Design review of the part built by this model. Coordinates are the model's own, in mm. A direction names the side the tool comes from. Give positions to 0.01 mm unless a question says otherwise; leave off trailing zeros. Loops run counter-clockwise (first coordinate to the right, second up) from the corner with the lowest first, then second, coordinate; pieces in that order, holes last. Notation, with made-up numbers: (-7.5, -40) -> (43.5, -40) arc R22 cw to (43.5, -11) -> close; hole circle Ø9 at (-25.5, 65). An arc over 180 degrees is marked (long way). Answer in a Markdown table with one row per item. Add a question column.
(1) For faces 1 (the flat face through (22.67, -1150.66, 35.4)), 2 (the flat face through (23.09, -1150.66, 36.52)), list the 3-axis set-ups (+Z, -Z, +X, -X, +Y, -Y) from which the entire face can be reached by the end or side of a thin tool; tool diameter is ignored.
(2) For pin 1 (11 mm diameter, centred on y = -1152.5, z = 5, fed in from +X); pin 2 (5 mm diameter, centred on y = -1213, z = 2.5, fed in from -X); pin 3 (2 mm diameter, centred on x = 13, y = -358.5, fed in from +Z), all flat-tipped, find the tip position at first contact; note any pin that passes through.
(3) Consider section B-B on x = 27.5. Write out the cut boundary in (y, z).
(4) For line 1 (X direction, y = -1862.5, z = 5.5); line 2 (X direction, y = -2009.5, z = 48); line 3 (Z direction, x = 58.5, y = -665), list the stretches that pass through material, from the lowest coordinate up.
(5) Consider section A-A on y = -1767. Write out the cut boundary in (x, z).
from build123d import *

# Parameters (mm, degrees)
F1_DEPTH = 2334


with BuildPart() as f1:
    # F0 (on Front) → F1 (new body)
    with BuildSketch(Plane.XZ):
        with BuildLine():
            Line((0, 10), (0, 0))
            Line((0, 0), (1, 0))
            Line((1, 0), (1, 10))
            ThreePointArc((1, 10), (0.414214, 11.414214), (-1, 12))
            Line((-1, 12), (-13, 12))
            ThreePointArc((-13, 12), (-13.707107, 12.292893), (-14, 13))
            Line((-14, 13), (-14, 26.397954))
            ThreePointArc((-14, 26.397954), (-13.780479, 27.023135), (-13.218295, 27.373836))
            Line((-13.218295, 27.373836), (59.579564, 43.657993))
            ThreePointArc((59.579564, 43.657993), (60.703931, 44.359395), (61.142973, 45.609759))
            Line((61.142973, 45.609759), (61.142973, 53.808736))
            Line((61.142973, 53.808736), (60.142973, 53.808736))
            Line((60.142973, 53.808736), (60.142973, 45.609759))
            ThreePointArc((60.142973, 45.609759), (59.923452, 44.984577), (59.361268, 44.633876))
            Line((59.361268, 44.633876), (-14.218295, 28.17486))
            ThreePointArc((-14.218295, 28.17486), (-14.780479, 27.824159), (-15, 27.198977))
            Line((-15, 27.198977), (-15, 12))
            ThreePointArc((-15, 12), (-14.707107, 11.292893), (-14, 11))
            Line((-14, 11), (-1, 11))
            ThreePointArc((-1, 11), (-0.292893, 10.707107), (0, 10))
        make_face()
    extrude(amount=F1_DEPTH)


solid = f1.part
Values follow:
| question | item | result |
|---|---|---|
| 1 | face 1 | +X, +Y, -Y |
| 1 | face 2 | +Z, -X, +Y, -Y |
| 2 | pin 1 | x = 1 |
| 2 | pin 2 | x = 0 |
| 2 | pin 3 | z = 34.49 |
| 3 | outline | (-2334, 36.48) -> (0, 36.48) -> (0, 37.51) -> (-2334, 37.51) -> close |
| 4 | line 1 | 0 to 1 |
| 4 | line 2 | 60.14 to 61.14 |
| 4 | line 3 | 43.42 to 44.44 |
| 5 | outline | (-15, 12) arc R1 ccw to (-14, 11) -> (-1, 11) arc R1 cw to (0, 10) -> (0, 0) -> (1, 0) -> (1, 10) arc R2 ccw to (-1, 12) -> (-13, 12) arc R1 cw to (-14, 13) -> (-14, 26.4) arc R1 cw to (-13.22, 27.37) -> (59.58, 43.66) arc R2 ccw to (61.14, 45.61) -> (61.14, 53.81) -> (60.14, 53.81) -> (60.14, 45.61) arc R1 cw to (59.36, 44.63) -> (-14.22, 28.17) arc R1 ccw to (-15, 27.2) -> close |
